```python
from build123d import *

# Parameters (mm, degrees)
F0_R     = 10
F0_R_2   = 5.5
F0_R_3   = 4.05
F1_DEPTH = 3.8
F2_DEPTH = 6.8
F3_SIZE  = 1.2
F4_DEPTH = 4.2
F6_DEPTH = 1
F7_SIZE2 = 0.5
F7_SIZE  = 0.5


with BuildPart() as f1:
    # F0 (on Top) → F1 (new body)
    with BuildSketch(Plane.XY):
        Circle(F0_R)
        Circle(F0_R_2, mode=Mode.SUBTRACT)
        Circle(F0_R_3)
        Circle(F0_R_2)
        Circle(F0_R_3, mode=Mode.SUBTRACT)
    extrude(amount=F1_DEPTH)

    # F0 (on Top) → F2 (join)
    with BuildSketch(Plane.XY):
        Circle(F0_R_3)
    extrude(amount=F2_DEPTH)

    # F3
    f3_edges = [f1.edges().sort_by_distance(p)[0] for p in [
        (-10, 0, 3.8),
    ]]
    chamfer(f3_edges, length=F3_SIZE)

    # F0 (on Top) → F4 (join)
    with BuildSketch(Plane.XY):
        Circle(F0_R_2)
        Circle(F0_R_3, mode=Mode.SUBTRACT)
    extrude(amount=F4_DEPTH)

    # F5 (on face) → F6 (cut)
    with BuildSketch(Plane(origin=(0, 0, 0), x_dir=(1, 0, 0), z_dir=(0, 0, -1))):
        with BuildLine():
            ThreePointArc((0, 0), (-1.755002, 5), (0, 10))
            ThreePointArc((0, 10), (-0.648262, 9.978966), (-1.293797, 9.915951))
            ThreePointArc((-1.293797, 9.915951), (-2.744355, 4.562366), (-0.780625, -0.625))
            ThreePointArc((-0.780625, -0.625), (0.745504, -5.364534), (-1.265312, -9.919626))
            ThreePointArc((-1.265312, -9.919626), (-0.633931, -9.979886), (0, -10))
            ThreePointArc((0, -10), (1.755002, -5), (0, 0))
        make_face()
        with BuildLine():
            ThreePointArc((1.265312, 9.919626), (0.633931, 9.979886), (0, 10))
            ThreePointArc((0, 10), (-1.755002, 5), (0, 0))
            Line((0, 0), (1.238317, 0))
            ThreePointArc((1.238317, 0), (1.016198, 0.317427), (0.780625, 0.625))
            ThreePointArc((0.780625, 0.625), (-0.745504, 5.364534), (1.265312, 9.919626))
        make_face()
        with BuildLine():
            Line((1.238317, 0), (0, 0))
            ThreePointArc((0, 0), (1.755002, -5), (0, -10))
            ThreePointArc((0, -10), (0.648262, -9.978966), (1.293797, -9.915951))
            ThreePointArc((1.293797, -9.915951), (2.754861, -4.949646), (1.238317, 0))
        make_face()
    extrude(amount=-F6_DEPTH, mode=Mode.SUBTRACT)

    # F7
    f7_edges = [f1.edges().sort_by_distance(p)[0] for p in [
        (-2.744355, -4.562366, 0),
        (0.745504, 5.364534, 0),
        (2.744355, 4.562366, 0),
        (-0.745504, -5.364534, 0),
    ]]
    chamfer(f7_edges, length=F7_SIZE, length2=F7_SIZE2)


solid = f1.part
```
Design review of the part built by this model. Coordinates are the model's own, in mm. A direction names the side the tool comes from. Round coordinates to 2 decimals unless told otherwise and drop trailing zeros. Order: outer loops, then holes, each group sorted by start corner. A loop starts at its lowest first (then second) coordinate and runs counter-clockwise, first axis right, second up. Notation, with made-up numbers: (9, -10.5) - (57, -10.5) arc R8 cw to (57, 4.5) - close; hole circle Ø9 at (-17, 60). An arc over 180 degrees is marked (long way). Return JSON: item names as keys, results as strings.
Q1. For pin 1 Ø1 at (x, z) = (8, 5) entering from +Y; pin 2 Ø2 at (x, y) = (7, 4.5) entering from +Z; pin 3 Ø1 at (y, z) = (-1, 1) entering from +X; pin 4 Ø4 at (x, y) = (2, 5) entering from +Z, all flat-tipped, find the tip position at first contact; note any pin that passes through.
Computed values:
{"pin 1": "passes through", "pin 2": "stops at z = 3.8", "pin 3": "stops at x = 9.99", "pin 4": "stops at z = 6.8"}
Q2. Consider section B-B on z = 1.5. Write out the cut boundary in (x, y).
Computed values:
{"outline": "circle Ø20 at (0, 0)"}
Q3. The part is to be moulded in two halves that separate along X. For faces 4 (the cylindrical face through (-2.17, -9.76, 1.28)), 5 (the cylindrical face through (-2.748, -4.641, 0.746)), 6 (the flat face through (5, 0, 0)), 7 (the cylindrical face through (2.755, 5.023, 0.746)), say which applies: pulls with the +X half, pulls with the -X half, needs draft (parallel to the pull), parting line crosses it, or undercut.
Computed values:
{"face 4": "parting line crosses it", "face 5": "undercut", "face 6": "needs draft", "face 7": "undercut"}
Q4. Consider section A-A on z = 3. Write out the cut boundary in (x, y).
Computed values:
{"outline": "circle Ø19.2 at (0, 0)"}
Q5. Machinability: for faces 1 (the flat face through (0, 0, 6.8)), 2 (the cylindrical face through (-0.75, -5.29, 0.75)), 3 (the cylindrical face through (-0.878, -3.954, 5.482)), which of the approach directions +Z, -Z, +X, -X, +Y, -Y give a long, thin tool a straight path to every point of the face, cutting with its end or side? Answer none if there is none.
Computed values:
{"face 1": "+Z, +X, -X, +Y, -Y", "face 2": "-Z", "face 3": "+Z"}
Q6. Wall thickness on L1, parallel to Z at x = 0.5, y = -0.75; L2, parallel to X at y = -3.5, z = 0.75; L3, parallel to Z at x = 3, y = -4.75: over which ranges is each line inside the solid? List them lowest first. Write a range as [from, to].
Computed values:
{"L1": "z = [1, 6.8]", "L2": "x = [-9.37, -2.63], [-0.59, 9.37]", "L3": "z = [0, 3.8]"}
